The model under review builds one solid part; all positions refer to its coordinate system, in mm. A direction names the side the tool comes from. Give positions to 0.01 mm unless a question says otherwise; leave off trailing zeros. Write each loop counter-clockwise with the first axis right and the second up, starting at its lowest first coordinate (ties: lowest second). Pieces come first, ordered by that corner, then holes. Notation, with made-up numbers: (-8.75, 48.25) -> (5.25, 48.25) arc R18 ccw to (5.25, 54.25) -> close; hole circle Ø9 at (72, -27.5). An arc over 180 degrees is marked (long way). Use CSV: the item, a comma, the result in double quotes.
```python
from build123d import *

# Parameters (mm, degrees)
SKETCH_1_W           = 40
SKETCH_1_H           = 94
EXTRUDE_1_DEPTH      = 4
EXTRUDE_2_DEPTH      = 47
EXTRUDE_2_DEPTH_BACK = 47
SKETCH_2_R           = 2.1
SKETCH_3_W           = 11
SKETCH_3_H           = 24.75
CUT_EXTRUDE_1_DEPTH  = 14
SKETCH_4_R           = 2
CUT_EXTRUDE_2_DEPTH  = 14
CHAMFER_2_SIZE       = 1.5
FILLET_1_R           = 2


with BuildPart() as part:
    # Эскиз1 → Бобышка-Вытянуть1 (new body)
    with BuildSketch(Plane(origin=(0, 0, 0), x_dir=(1, 0, 0), z_dir=(0, 1, 0))):
        Rectangle(SKETCH_1_W, SKETCH_1_H)
    extrude(amount=EXTRUDE_1_DEPTH)

    # Эскиз2 → Бобышка-Вытянуть2 (add, two sides: drawn at the far end of the back side and taken through both)
    with BuildSketch(Plane.XY.offset(-EXTRUDE_2_DEPTH_BACK)):
        with BuildLine():
            Line((-20, 0), (-25.5, 0))
            ThreePointArc((-25.5, 0), (-28.81662479, 9.887482194), (-20.208497378, 4))
            Line((-20.208497378, 4), (-20, 4))
            Line((-20, 4), (-20, 0))
        make_face()
        with Locations(Location((-25.5, 5.5, 0), (0, 0, 180))):
            Circle(SKETCH_2_R, mode=Mode.SUBTRACT)
    extrude(amount=EXTRUDE_2_DEPTH + EXTRUDE_2_DEPTH_BACK)

    # Эскиз3 → Вырез-Вытянуть1 (cut)
    with BuildSketch(Plane(origin=(0, 0, 0), x_dir=(1, 0, 0), z_dir=(0, 1, 0))):
        with Locations((-25.5, 19.825)):
            Rectangle(SKETCH_3_W, SKETCH_3_H)
        with Locations((-25.5, -19.825)):
            Rectangle(SKETCH_3_W, SKETCH_3_H)
    extrude(amount=CUT_EXTRUDE_1_DEPTH, mode=Mode.SUBTRACT)

    # Эскиз4 → Вырез-Вытянуть2 (cut)
    with BuildSketch(Plane(origin=(0, 4, 0), x_dir=(1, 0, 0), z_dir=(0, 1, 0))):
        with Locations(Location((-5, 32, 0), (0, 0, 270))):
            Circle(SKETCH_4_R)
        with Locations(Location((-5, -32, 0), (0, 0, 270))):
            Circle(SKETCH_4_R)
    extrude(amount=-CUT_EXTRUDE_2_DEPTH, mode=Mode.SUBTRACT)

    # Фаска2
    chamfer_2_edges = [part.edges().sort_by_distance(p)[0] for p in [
        (-5, 4, -34),
        (-5, 4, 30),
    ]]
    chamfer(chamfer_2_edges, length=CHAMFER_2_SIZE)

    # Скругление1
    fillet_1_edges = [part.edges().sort_by_distance(p)[0] for p in [
        (20, 4, 0),
    ]]
    fillet(fillet_1_edges, radius=FILLET_1_R)


solid = part.part
```
Q1. Machinability: for faces 4 (the flat face through (-23, 5, 32.2)), 5 (the cylindrical face through (-27.503, 4.869, 39.496)), which of the approach directions +Z, -Z, +X, -X, +Y, -Y give a long, thin tool a straight path to every point of the face, cutting with its end or side? Answer none if there is none.
Derived:
face 4,"-X, +Y, -Y"
face 5,"+Z, -Z"
Q2. The part is to be moulded in two halves that separate along Y. For faces 1 (the flat face through (-2, 0, -1)), 2 (the cylindrical face through (-27.503, 4.869, -39.704)), 3 (the flat face through (-11, 3, 47)), say which applies: pulls with the +Y half, pulls with the -Y half, needs draft (parallel to the pull), parting line crosses it, or undercut.
Derived:
face 1,"pulls with the -Y half"
face 2,"undercut"
face 3,"needs draft"
Q3. Insertion check: pin 1 (4.5 mm diameter, centred on y = 3, z = -16, fed in from -X); pin 2 (8 mm diameter, centred on x = 10.5, z = 6, fed in from +Y). Each pin has a flat end and moves straight along its axis. Give the tip position at first contact, or say it passes through.
Derived:
pin 1,"stops at x = -20"
pin 2,"stops at y = 4"
Q4. Consider section C-C (y = 9.5). Write out the cut boundary in (x, z).
Derived:
outline,"(-29.27, -47) -> (-21.73, -47) -> (-21.73, -32.2) -> (-29.27, -32.2) -> close; (-29.27, -7.45) -> (-21.73, -7.45) -> (-21.73, 7.45) -> (-29.27, 7.45) -> close; (-29.27, 32.2) -> (-21.73, 32.2) -> (-21.73, 47) -> (-29.27, 47) -> close"
Q5. Consider section B-B (x = -5). Write out the cut boundary in (y, z).
Derived:
outline,"(0, -47) -> (4, -47) -> (4, -35.5) -> (2.5, -34) -> (0, -34) -> close; (0, -30) -> (2.5, -30) -> (4, -28.5) -> (4, 28.5) -> (2.5, 30) -> (0, 30) -> close; (0, 34) -> (2.5, 34) -> (4, 35.5) -> (4, 47) -> (0, 47) -> close"
Q6. To check wall thickness, follow probe 1 along Z at (x, y) = (-23.5, 4); probe 2 along X at (y, z) = (5.5, 40.5). State the ranges of each line that lie inside material, in increasing order.
Derived:
probe 1,"z = -47 to -32.2, -7.45 to 7.45, 32.2 to 47"
probe 2,"x = -31 to -27.6, -23.4 to -20"
Q7. Consider section D-D (z = 1). Write out the cut boundary in (x, y).
Derived:
outline,"(-25.5, 0) -> (20, 0) -> (20, 2) arc R2 ccw to (18, 4) -> (-20.21, 4) arc R5.5 ccw (long way) to start; hole circle Ø4.2 at (-25.5, 5.5)"
Q8. Consider section A-A (y = 5.5). Write out the cut boundary in (x, z).
Derived:
outline,"(-31, -47) -> (-27.6, -47) -> (-27.6, -32.2) -> (-31, -32.2) -> close; (-31, -7.45) -> (-27.6, -7.45) -> (-27.6, 7.45) -> (-31, 7.45) -> close; (-31, 32.2) -> (-27.6, 32.2) -> (-27.6, 47) -> (-31, 47) -> close; (-23.4, -47) -> (-20, -47) -> (-20, -32.2) -> (-23.4, -32.2) -> close; (-23.4, -7.45) -> (-20, -7.45) -> (-20, 7.45) -> (-23.4, 7.45) -> close; (-23.4, 32.2) -> (-20, 32.2) -> (-20, 47) -> (-23.4, 47) -> close"
